Autodesk Inventor part; units mm, degrees
ref_plane "YZ Plane" through (0, 0, 0) normal (1, 0, 0) x (0, 1, 0)
ref_plane "XZ Plane" through (0, 0, 0) normal (0, 1, 0) x (-1, 0, 0)
ref_plane "XY Plane" through (0, 0, 0) normal (0, 0, 1) x (1, 0, 0)
sketch "Sketch7" plane through (0, 0, 0) normal (0, 0, 1) x (1, 0, 0)
  line L0 (182.5, 316.099272) -> (365, 0)
  line L1 (365, 0) -> (182.5, -316.099272)
  line L2 (182.5, -316.099272) -> (-182.5, -316.099272)
  line L3 (-182.5, -316.099272) -> (-365, 0)
  line L4 (-365, 0) -> (-182.5, 316.099272)
  line L5 (-182.5, 316.099272) -> (182.5, 316.099272)
  line L6 (0, 0) -> (-182.5, 316.099272)
  line L7 (0, 0) -> (365, 0)
  line L8 (0, 0) -> (0, 100)
  line L9 (0, 0) -> (100, 0) construction
  dimension "d56" = 365
  dimension "d69" = 100
  dimension "d70" = 90
  dimension "d71" = 30
extrude "Extrusion6" add sketch "Sketch7" along normal blind 3 contours L0 L7 L6 L5
sketch "Sketch8" plane through (0, 0, 3) normal (0, 0, 1) x (1, 0, 0)
  line L0 (37.655445, -30.221143) -> (-7.344555, 47.721143)
  line L1 (-7.344555, 47.721143) -> (-37.655445, 30.221143)
  line L2 (-37.655445, 30.221143) -> (7.344555, -47.721143)
  line L3 (7.344555, -47.721143) -> (37.655445, -30.221143)
  line L4 (37.655445, -30.221143) -> (-37.655445, 30.221143) construction
  line L5 (-7.344555, 47.721143) -> (7.344555, -47.721143) construction
  line L6 (37.655445, -30.221143) -> (127.655445, -30.221143) construction
  line L7 (-45, 17.5) -> (45, 17.5)
  line L8 (45, 17.5) -> (45, -17.5)
  line L9 (45, -17.5) -> (-45, -17.5)
  line L10 (-45, -17.5) -> (-45, 17.5)
  line L11 (-182.5, 316.099272) -> (0, 0)
  line L12 (-45, 17.5) -> (45, -17.5) construction
  line L13 (45, 17.5) -> (-45, -17.5) construction
  line L14 (-45, 17.5) -> (45, 17.5) construction
  dimension "d60" = 90
  dimension "d61" = 120
  dimension "d62" = 35
  dimension "d63" = 90
  dimension "d64" = 0
  dimension "d65" = 35
extrude "Extrusion7" cut sketch "Sketch8" against normal blind 3
sketch "Sketch9" plane through (0, 0, 3) normal (0, 0, 1) x (1, 0, 0)
  line L0 (0, 0) -> (152.5, 264.137748)
  line L1 (0, 0) -> (305, 0) construction
  line L2 (152.5, 264.137748) -> (163.75833, 257.637748)
  line L3 (152.5, 264.137748) -> (165.5, 264.137748) construction
  circle A0 centre (163.75833, 257.637748) radius 1.75
  line L4 (163.75833, 257.637748) -> (153.75833, 240.31724)
  circle A1 centre (153.75833, 240.31724) radius 1.75
  dimension "d72" = 305
  dimension "d73" = 60
  dimension "d74" = 13
  dimension "d75" = 30
  dimension "d76" = 3.5
  dimension "d77" = 20
  dimension "d78" = 90
  dimension "d79" = 3.5
extrude "Extrusion8" cut sketch "Sketch9" against normal blind 3
fillet "Fillet1" radius 5 3 edges at (182.5, 316.0993, 1.5) (365, 0, 1.5) (-182.5, 316.0993, 1.5)
fillet "Fillet2" radius 2 2 edges at (45, 17.5, 1.5) (-7.3446, 47.7211, 1.5)
fillet "Fillet3" radius 2 2 edges at (45, 0, 1.5) (10.1036, 17.5, 1.5)
fillet "Fillet4" radius 2 1 edges at (-22.5, 38.9711, 1.5)
sketch "Sketch13" plane through (0, 0, 3) normal (0, 0, 1) x (1, 0, 0)
  line L0 (-178.169873, 308.599272) -> (-23.5, 40.703194)
  line L1 (-23.5, 40.703194) -> (-28.5, 49.363448)
  line L2 (-28.5, 49.363448) -> (-80, 138.564065)
  line L3 (-80, 138.564065) -> (-88.660254, 133.564065)
  line L4 (-88.660254, 133.564065) -> (-37.160254, 44.363448)
  line L5 (-37.160254, 44.363448) -> (-28.5, 49.363448)
  line L6 (-28.5, 49.363448) -> (74.5, 49.363448) construction
  line L7 (47, 0) -> (356.339746, 0)
  line L8 (47, 0) -> (162, 0)
  line L9 (162, 0) -> (342, 0)
  line L10 (342, 0) -> (342, -10)
  line L11 (342, -10) -> (162, -10)
  line L12 (162, -10) -> (162, 0)
  point P0 (0, 0)
  dimension "d123" = 10
  dimension "d124" = 103
  dimension "d125" = 120
  dimension "d126" = 10
  dimension "d127" = 115
  dimension "d128" = 180
  dimension "d129" = 10
extrude "Extrusion12" add sketch "Sketch13" against normal blind 3
sketch "Sketch14" plane through (0, 0, 3) normal (0, 0, 1) x (1, 0, 0)
  line L0 (-178.169873, 308.599272) -> (-80, 138.564065)
  line L1 (-80, 138.564065) -> (-80, 138.564065)
  line L2 (-80, 138.564065) -> (-172, 297.912739)
  line L3 (-172, 297.912739) -> (-162.473721, 303.412739)
  line L4 (-162.473721, 303.412739) -> (-70.473721, 144.064065)
  line L5 (-70.473721, 144.064065) -> (-80, 138.564065)
  line L6 (47, 0) -> (162, 0)
  line L7 (47, 0) -> (56, 0)
  line L8 (56, 0) -> (162, 0)
  line L9 (162, 0) -> (162, 11)
  line L10 (162, 11) -> (56, 11)
  line L11 (56, 11) -> (56, 0)
  point P0 (0, 0)
  dimension "d132" = 0
  dimension "d133" = 184
  dimension "d134" = 11
  dimension "d135" = 9
  dimension "d136" = 106
  dimension "d137" = 11
extrude "Extrusion13" cut sketch "Sketch14" against normal blind 3
sketch "Sketch15" plane through (0, 0, 3) normal (0, 0, 1) x (1, 0, 0)
  line L0 (342, 0) -> (342, -10)
  line L1 (342, 0) -> (292, 0)
  circle A0 centre (292, 0) radius 2.75
  circle A1 centre (242, 0) radius 2.75
  circle A2 centre (192, 0) radius 2.75
  line L2 (-28.5, 49.363448) -> (-37.160254, 44.363448)
  line L3 (-28.5, 49.363448) -> (-46, 79.674337)
  line L4 (-28.5, 49.363448) -> (6.5, 49.363448) construction
  circle A3 centre (-46, 79.674337) radius 2.75
  circle A4 centre (-63.5, 109.985226) radius 2.75
  point P0 (0, 0)
  dimension "d140" = 50
  dimension "d141" = 5.5
  dimension "d144" = 50
  dimension "d149" = 35
  dimension "d150" = 120
  dimension "d151" = 5.5
  dimension "d154" = 35
extrude "Extrusion14" cut sketch "Sketch15" against normal blind 3
sketch "Sketch16" plane through (0, 0, 0) normal (0, 0, -1) x (-1, 0, 0)
  line L0 (181.006538, 319.907407) -> (181.006538, -10.092593)
  line L1 (181.006538, -10.092593) -> (-363.993462, -10.092593)
  line L2 (-363.993462, -10.092593) -> (-363.993462, 319.907407)
  line L3 (-363.993462, 319.907407) -> (181.006538, 319.907407)
  line L4 (-342, -10) -> (-162, -10)
  point P0 (0, 0)
  dimension "d161" = 545
  dimension "d162" = 330
properties part number "Acrylic_top"
Part model, mm, in its own coordinate system. Round coordinates to 2 decimals unless told otherwise and drop trailing zeros. Write each loop counter-clockwise with the first axis right and the second up, starting at its lowest first coordinate (ties: lowest second). Pieces come first, ordered by that corner, then holes. Notation, with made-up numbers: M 87.5,11.5 L 131.5,11.5 A27 ccw 131.5,41.5 Z; hole C 45,77 d6. An arc over 180 degrees is marked long. Return JSON: item names as keys, results as strings. Group by question number.
(1) Two-plate mould, pull along X, no slides. Class faces 1 (the face through (-63.27, 89.59, 1.52)), 2 (the face through (1.702, 32.052, 1.521)), 3 (the face through (271.07, 162.69, 1.48)): +X half, -X half, draft (parallel to the pull), parting line (faces both ways), or undercut.
(2) Saw through at C-C on z = 2.3. Count the separate pieces of the cut face and the enclosed holes in it, then the cut area to 3 significant figures.
(3) Pin check, flat tips, straight feed: pin 1 Ø0.9 at (y, z) = (-1.5, 1.5) entering from -X; pin 2 Ø3 at (x, y) = (153.76, 240.32) entering from -Z; pin 3 Ø0.9 at (y, z) = (7, 1.5) entering from +X; pin 4 Ø1.5 at (x, z) = (347.5, 1) entering from -Y. Stop position of each tip, or through.
(4) Drill centre lines: probe 1 along Y at (x, z) = (292.5, 1.8); probe 2 along Y at (x, z) = (144.5, 0.9); probe 3 along Y at (x, z) = (49, 0.5). Where is each one in solid material? Low to high.
(5) Saw through at A-A on x = 140.5. Write the cut outline in (y, z), then the cut area to 3 significant figures.
(6) Saw through at B-B on y = 219. Write the cut outline in (x, z), then the cut area to 3 significant figures.
Returned:
{
 "1": {"face 1": "-X half", "face 2": "undercut", "face 3": "+X half"},
 "2": {"separate pieces": "1", "enclosed holes": "7", "area": "113,000 mm²"},
 "3": {"pin 1": "x = 162", "pin 2": "through", "pin 3": "x = 361.09", "pin 4": "y = 0"},
 "4": {"probe 1": "-10 to -2.7, 2.7 to 125.57", "probe 2": "11 to 316.1", "probe 3": "0 to 316.1"},
 "5": {"outline": "M 11,0 L 316.1,0 L 316.1,3 L 11,3 Z", "area": "915 mm²"},
 "6": {"outline": "M -113.74,0 L 238.56,0 L 238.56,3 L -113.74,3 Z", "area": "1,060 mm²"}
}
